from build123d import *

# Parameters (mm, degrees)
SKETCH_1_W          = 6.2
SKETCH_1_H          = 12
EXTRUDE_1_DEPTH     = 40
SKETCH_2_R          = 2.5
CUT_EXTRUDE_1_DEPTH = 41.919921799
SKETCH_3_R          = 2.5
EXTRUDE_2_DEPTH     = 170


with BuildPart() as part:
    # 草图1 → 凸台-拉伸1 (new body)
    with BuildSketch(Plane.XY):
        Rectangle(SKETCH_1_W, SKETCH_1_H)
    extrude(amount=EXTRUDE_1_DEPTH)

    # 草图2 → 切除-拉伸1 (cut, through all)
    with BuildSketch(Plane(origin=(3.1, 0, 0), x_dir=(0, 0, -1), z_dir=(1, 0, 0))):
        with Locations((-34, 0)):
            Circle(SKETCH_2_R)
    extrude(amount=-CUT_EXTRUDE_1_DEPTH, mode=Mode.SUBTRACT)

    # 草图3 → 凸台-拉伸2 (add)
    with BuildSketch(Plane(origin=(0, 0, 0), x_dir=(-1, 0, 0), z_dir=(0, 0, -1))):
        Circle(SKETCH_3_R)
    extrude(amount=EXTRUDE_2_DEPTH)


solid = part.part
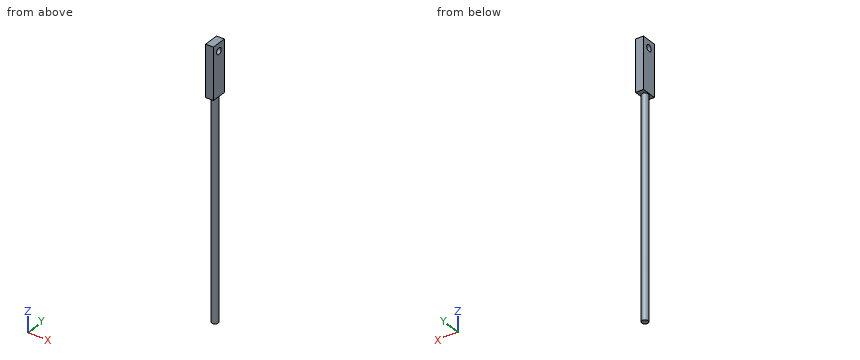
Geometry: final body of the model. Coordinates: model frame, mm. Round coordinates to 2 decimals unless told otherwise and drop trailing zeros. Order: outer loops, then holes, each group sorted by start corner. A loop starts at its lowest first (then second) coordinate and runs counter-clockwise, first axis right, second up. Notation, with made-up numbers: (-26, 9.25) -> (16, 9.25) arc R16 ccw to (16, 17.25) -> close; hole circle Ø5 at (16, 25.25). An arc over 180 degrees is marked (long way). Put each result on its own line as item: value. Start each with the question number.
Q1. Section D-D on z = -84. Return the cut outline in (x, y).
Q2. Section A-A on y = 0. Return the cut outline in (x, z).
Q3. Section B-B on z = 34. Return the cut outline in (x, y).
Q4. Line query: probe 1 along Y at (x, z) = (0.25, 34); probe 2 along Z at (x, y) = (-2.5, -4.25); probe 3 along Z at (x, y) = (2.25, -2). Output: solid intervals per line, ascending.
Q5. First-contact query: pin 1 (6 mm diameter, centred on y = -3.5, z = -4, fed in from -X); pin 2 (1 mm diameter, centred on x = 2, z = -36.5, fed in from -Y); pin 3 (4.5 mm diameter, centred on y = 0, z = 34, fed in from -X). Flat tips, straight axial feed; report the tip coordinate or a pass-through.
Q6. Section C-C on x = 0. Return the cut outline in (y, z).
Ans:
1. outline: circle Ø5 at (0, 0)
2. outline: (-3.1, 0) -> (-2.5, 0) -> (-2.5, -170) -> (2.5, -170) -> (2.5, 0) -> (3.1, 0) -> (3.1, 31.5) -> (-3.1, 31.5) -> close; (-3.1, 36.5) -> (3.1, 36.5) -> (3.1, 40) -> (-3.1, 40) -> close
3. outline: (-3.1, -6) -> (3.1, -6) -> (3.1, -2.5) -> (-3.1, -2.5) -> close; (-3.1, 2.5) -> (3.1, 2.5) -> (3.1, 6) -> (-3.1, 6) -> close
4. probe 1: y = -6 to -2.5, 2.5 to 6
4. probe 2: z = 0 to 40
4. probe 3: z = 0 to 32.5, 35.5 to 40
5. pin 1: stops at x = -2.45
5. pin 2: stops at y = -2
5. pin 3: passes through
6. outline: (-6, 0) -> (-2.5, 0) -> (-2.5, -170) -> (2.5, -170) -> (2.5, 0) -> (6, 0) -> (6, 40) -> (-6, 40) -> close; hole circle Ø5 at (0, 34)
